Geometry check sheet. Reference: drawing and pictorial views, mm from the part's lowest x, y, z. Round coordinates to 2 decimals unless told otherwise and drop trailing zeros. Order: outer loops, then holes, each group sorted by start corner. A loop starts at its lowest first (then second) coordinate and runs counter-clockwise, first axis right, second up. Notation, with made-up numbers: (1.25, 33.5) -> (29.25, 33.5) arc R8 cw to (29.25, 37.5) -> close; hole circle Ø6 at (-30.75, 47.5). An arc over 180 degrees is marked (long way). Put each result on its own line as item: value.
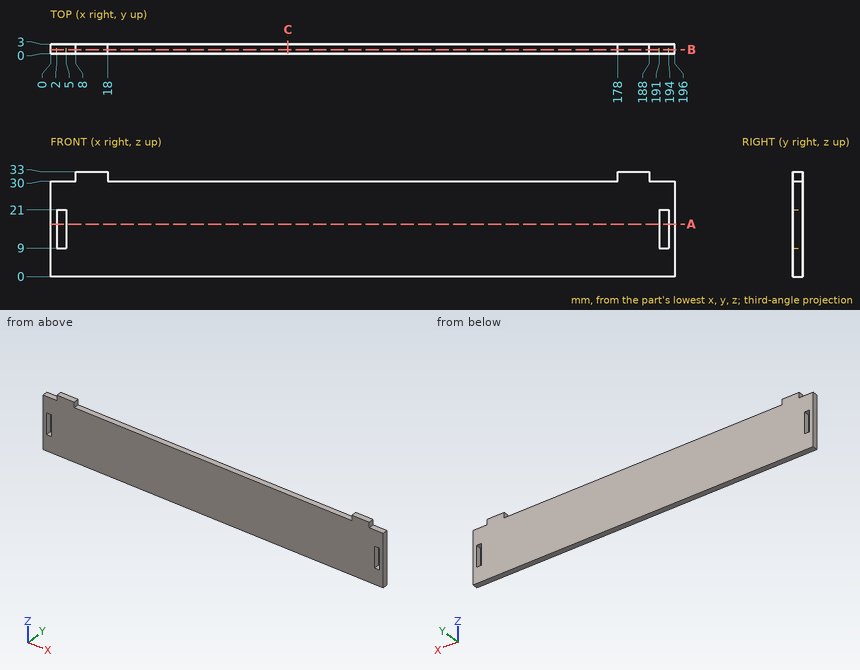
Item 1: Sectioned sample at B-B, the plane y = 1.2. Record the boundary of the cut face in (x, z).
Geometry check:
outline: (0, 0) -> (196, 0) -> (196, 30) -> (188, 30) -> (188, 33) -> (178, 33) -> (178, 30) -> (18, 30) -> (18, 33) -> (8, 33) -> (8, 30) -> (0, 30) -> close; hole (2, 9) -> (5, 9) -> (5, 21) -> (2, 21) -> close; hole (191, 9) -> (194, 9) -> (194, 21) -> (191, 21) -> close
Item 2: Material ranges on line 1 along X through (y, z) = (2.2, 14.5); line 2 along Z through (x, y) = (118, 0.8), recorded low to high.
Geometry check:
line 1: 0 to 2, 5 to 191, 194 to 196
line 2: 0 to 30
Item 3: Sectioned sample at C-C, the plane x = 74.5. Record the boundary of the cut face in (y, z), then the cut area to 3 significant figures.
Geometry check:
outline: (0, 0) -> (3, 0) -> (3, 30) -> (0, 30) -> close
area: 90.0 mm2
Item 4: Depth check by flat-ended pin: pin 1 Ø0.9 at (y, z) = (2, 32) entering from -X; pin 2 Ø1.5 at (x, y) = (193, 1) entering from +Z; pin 3 Ø1.5 at (y, z) = (2, 31.5) entering from +X. Enter the tip coordinate at first touch or a pass-through.
Geometry check:
pin 1: x = 8
pin 2: z = 30
pin 3: x = 188
Item 5: Sectioned sample at A-A, the plane z = 16.5. Record the boundary of the cut face in (x, y).
Geometry check:
outline: (0, 0) -> (2, 0) -> (2, 3) -> (0, 3) -> close; (5, 0) -> (191, 0) -> (191, 3) -> (5, 3) -> close; (194, 0) -> (196, 0) -> (196, 3) -> (194, 3) -> close
